Input: dimensioned drawing with shaded views. Units: mm. Origin: part minimum x, y, z. Give positions to 0.01 mm unless a question says otherwise; leave off trailing zeros. Order: outer loops, then holes, each group sorted by start corner. A loop starts at its lowest first (then second) coordinate and runs counter-clockwise, first axis right, second up.
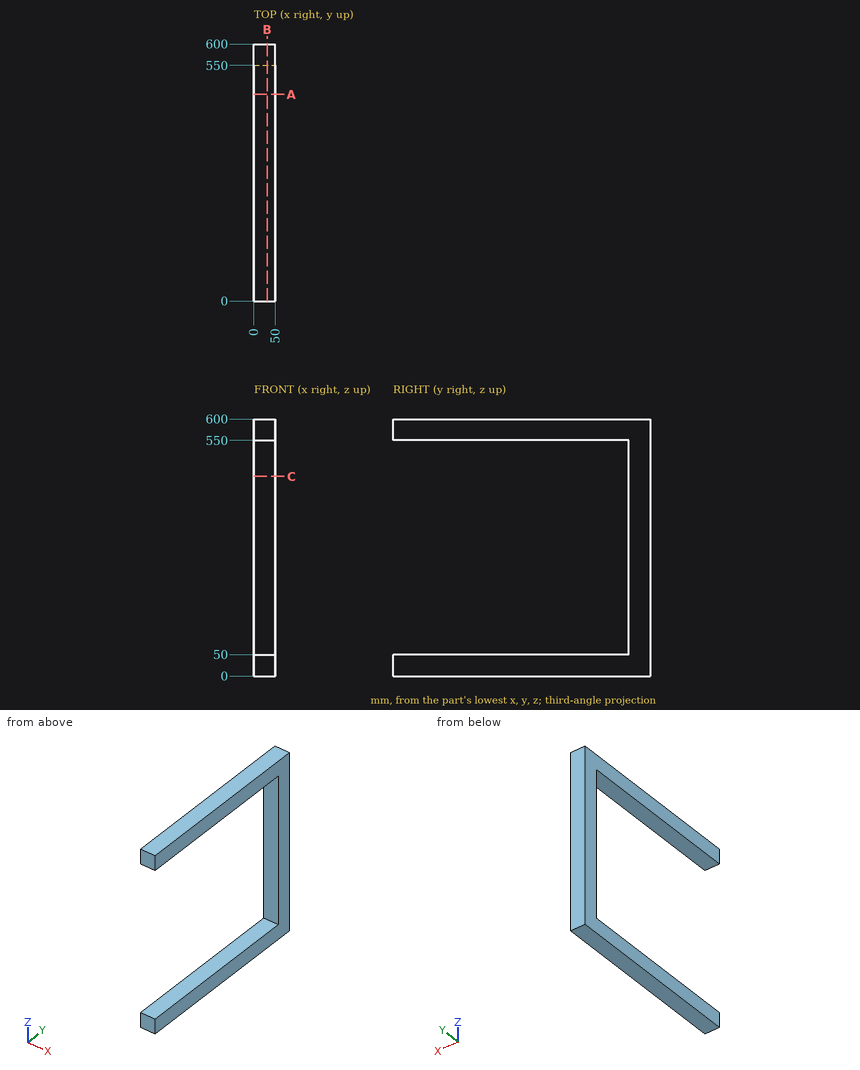
1) Section query C-C, the plane z = 466. Return the cut outline in (x, y), and give its area (3 significant figures).
Report:
outline: (0, 550) - (50, 550) - (50, 600) - (0, 600) - close
area: 2,500 mm2
2) Pin query (flat end, axial travel): pin 1 (12 mm diameter, centred on x = 12.5, z = 75.5, fed in from -Y); pin 2 (12 mm diameter, centred on x = 30.5, y = 311, fed in from -Z). Return the tip coordinate at first contact, or that it passes through.
Report:
pin 1: stops at y = 550
pin 2: stops at z = 0
3) Section query B-B, the plane x = 31. Return the cut outline in (y, z), and give its area (3 significant figures).
Report:
outline: (0, 0) - (600, 0) - (600, 600) - (0, 600) - (0, 550) - (550, 550) - (550, 50) - (0, 50) - close
area: 85,000 mm2
4) Material intervals for L1, parallel to Z at x = 22, y = 392.5; L2, parallel to Y at x = 3.5, z = 137.5, sorted ascending.
Report:
L1: z = 0 to 50, 550 to 600
L2: y = 550 to 600
5) Section query A-A, the plane y = 482.5. Return the cut outline in (x, z).
Report:
outline: (0, 0) - (50, 0) - (50, 50) - (0, 50) - close; (0, 550) - (50, 550) - (50, 600) - (0, 600) - close
